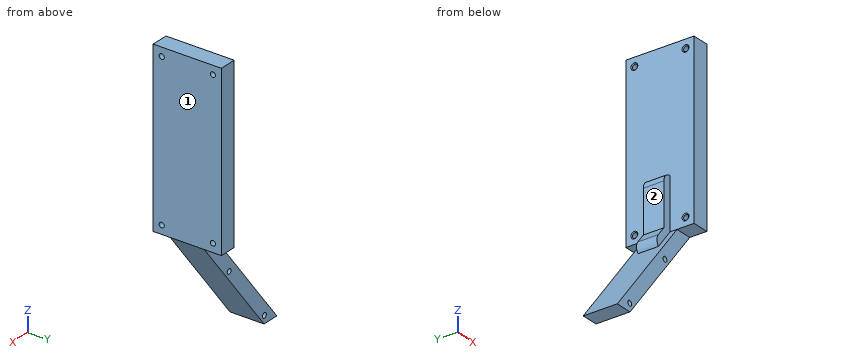
```python
from build123d import *

# Parameters (mm, degrees)
SKETCH_1_W           = 100
SKETCH_1_H           = 40
EXTRUDE_1_DEPTH      = 10
EXTRUDE_2_DEPTH      = 30
SKETCH_4_R           = 1.5
CUT_EXTRUDE_1_DEPTH  = 127.085153879
CUT_EXTRUDE_2_DEPTH  = 10
SKETCH_7_R           = 1.5
CUT_EXTRUDE_3_DEPTH  = 10
CHAMFER_2_SIZE       = 0.5
EXTRUDE_3_DEPTH      = 6
EXTRUDE_3_DEPTH_BACK = 6
FILLET_1_R           = 5


with BuildPart() as part:
    # 草图1 → 凸台-拉伸1 (new body)
    with BuildSketch(Plane(origin=(0, 0, 0), x_dir=(0, 0, -1), z_dir=(1, 0, 0))):
        Rectangle(SKETCH_1_W, SKETCH_1_H)
    extrude(amount=EXTRUDE_1_DEPTH)

    # 草图3 → 凸台-拉伸2 (add)
    with BuildSketch(Plane(origin=(0, 20, 0), x_dir=(1, 0, 0), z_dir=(0, 1, 0))):
        Polygon((10, 50), (-36.87713759, 110), (-46.87713759, 110), (0, 50), align=None)
    extrude(amount=-EXTRUDE_2_DEPTH)

    # 草图4 → 切除-拉伸1 (cut, through all)
    with BuildSketch(Plane(origin=(0, 20, 0), x_dir=(1, 0, 0), z_dir=(0, 1, 0))):
        with Locations(Location((-37.168406916, 105.5, 0), (0, 0, 270))):
            Circle(SKETCH_4_R)
        with Locations(Location((-9.463640527, 70.039516088, 0), (0, 0, 270))):
            Circle(SKETCH_4_R)
    extrude(amount=-CUT_EXTRUDE_1_DEPTH, mode=Mode.SUBTRACT)

    # 草图5 → 切除-拉伸2 (cut)
    with BuildSketch(Plane(origin=(0, 20, 0), x_dir=(1, 0, 0), z_dir=(0, 1, 0))):
        Polygon((10, 50), (0, 50), (-46.87713759, 110), (-36.87713759, 110), align=None)
    extrude(amount=-CUT_EXTRUDE_2_DEPTH, mode=Mode.SUBTRACT)

    # 草图7 → 切除-拉伸3 (cut)
    with BuildSketch(Plane(origin=(10, 0, 0), x_dir=(0, 0, -1), z_dir=(1, 0, 0))):
        with Locations((-45, 15)):
            Circle(SKETCH_7_R)
        with Locations((-45, -15)):
            Circle(SKETCH_7_R)
        with Locations((45, -15)):
            Circle(SKETCH_7_R)
        with Locations((45, 15)):
            Circle(SKETCH_7_R)
    extrude(amount=-CUT_EXTRUDE_3_DEPTH, mode=Mode.SUBTRACT)

    # 倒角2
    chamfer_2_edges = [part.edges().sort_by_distance(p)[0] for p in [
        (0, 15, -43.5),
        (0, -15, -43.5),
        (0, -15, 46.5),
        (0, 15, 46.5),
    ]]
    chamfer(chamfer_2_edges, length=CHAMFER_2_SIZE)

    # 草图9 → 凸台-拉伸3 (add, two sides: drawn at the far end of the back side and taken through both)
    with BuildSketch(Plane(origin=(0, 0, 0), x_dir=(1, 0, 0), z_dir=(0, 1, 0)).offset(-EXTRUDE_3_DEPTH_BACK)):
        Polygon((-9.23492213, 61.820161304), (-12.339726869, 59.394421988), (-5, 50), (-5, 20), (0, 20), (0, 50), align=None)
    extrude(amount=EXTRUDE_3_DEPTH + EXTRUDE_3_DEPTH_BACK)

    # 圆角1
    # the kernel refuses this fillet: 5 mm, written as the material it takes off along each edge
    with BuildSketch(Plane(origin=(-5, -18.5, -20), x_dir=(1, 0, 0), z_dir=(0, 1, 0))) as fillet_1_piece_1:
        with BuildLine():
            CenterArc((FILLET_1_R, FILLET_1_R), FILLET_1_R, 180, 90)
            Line((0, FILLET_1_R), (-FILLET_1_R * 0.02, FILLET_1_R))
            Line((-FILLET_1_R * 0.02, FILLET_1_R), (-FILLET_1_R * 0.02, -FILLET_1_R * 0.02))
            Line((-FILLET_1_R * 0.02, -FILLET_1_R * 0.02), (FILLET_1_R, -FILLET_1_R * 0.02))
            Line((FILLET_1_R, -FILLET_1_R * 0.02), (FILLET_1_R, 0))
        make_face()
    extrude(amount=37, mode=Mode.SUBTRACT)
    with BuildSketch(Plane(origin=(-12.339726869, -18.215899984, -59.394421988), x_dir=(0.7880107536067237, 0, -0.6156614753256561), z_dir=(0, 1, 0))) as fillet_1_piece_2:
        with BuildLine():
            CenterArc((5, -4.886359993), FILLET_1_R, 102.23895269, 77.76104731)
            Line((0, -4.886359993), (-0.1, -4.886359993))
            Line((-0.1, -4.886359993), (-0.1, 0))
            Line((-0.1, 0), (0, 0.1))
            ThreePointArc((0, 0.1), (1.970026884, 0.1), (3.918854843, 0.0977272))
            Line((3.918854843, 0.0977272), (3.940053768, 0))
        make_face()
    extrude(amount=36.431799967, mode=Mode.SUBTRACT)


solid = part.part
```
Verification items for the finished model (mm, model axes). Face numbers are marked on the shaded views. A direction names the side the tool comes from. Coordinates: 2 decimals unless noted, no trailing zeros. Order: outer loops, then holes, each group sorted by start corner. A loop starts at its lowest first (then second) coordinate and runs counter-clockwise, first axis right, second up. Notation, with made-up numbers: (7.5, 2) -> (51.5, 2) arc R29 ccw to (51.5, 23) -> close; hole circle Ø1 at (-8, 54). An arc over 180 degrees is marked (long way). Put each result on its own line as item: value. Start each with the question number.
1) Tool access check on the marked faces 1 and 2. Record the directions out of +Z, -Z, +X, -X, +Y, -Y that give a thin tool (end or side, any length) a straight path to the whole face; none if there is none.
2) Material ranges on L1, parallel to Y at x = 3, z = -45; L2, parallel to Z at x = 7.5, y = 10.5; L3, parallel to X at y = -2.5, z = -45.5, recorded low to high.
3) Cross-section at A-A (y = -15). Enter the section's corners in (x, z), plus the area to 4 significant figures.
4) Cross-section at D-D (z = -105.5). Enter the section's corners in (x, y), plus the area to 3 significant figures.
5) Go/stop test with flat-tipped pins: pin 1 (5 mm diameter, centred on y = -15, z = 45, fed in from -X); pin 2 (8 mm diameter, centred on x = -20.5, y = -6.5, fed in from -Z); pin 3 (3 mm diameter, centred on x = 4.5, y = 16, fed in from -Z); pin 4 (12 mm diameter, centred on x = -5.5, y = -1, fed in from +Z). Record where each tip stops, or that it passes through.
6) Cross-section at C-C (x = 2). Enter the section's corners in (y, z).
7) Cross-section at B-B (z = 45). Enter the section's corners in (x, y).
Geometry check:
1. face 1: +Z, -Z, +X, +Y, -Y
1. face 2: +Z, -X, +Y, -Y
2. L1: y = -20 to -16.5, -13.5 to 13.5, 16.5 to 20
2. L2: z = -50 to 50
2. L3: x = -5 to 10
3. outline: (0, -50) -> (10, -50) -> (10, -46.5) -> (0.5, -46.5) -> (0, -47) -> close; (0, -43) -> (0.5, -43.5) -> (10, -43.5) -> (10, 43.5) -> (0.5, 43.5) -> (0, 43) -> close; (0, 47) -> (0.5, 46.5) -> (10, 46.5) -> (10, 50) -> (0, 50) -> close
3. area: 939.5 mm^2
4. outline: (-43.36, -10) -> (-38.67, -10) -> (-38.67, 10) -> (-43.36, 10) -> close; (-35.67, -10) -> (-33.36, -10) -> (-33.36, 10) -> (-35.67, 10) -> close
4. area: 140 mm^2
5. pin 1: stops at x = 0
5. pin 2: stops at z = -94.16
5. pin 3: stops at z = -50
5. pin 4: stops at z = 50
6. outline: (-20, -50) -> (-10, -50) -> (-10, -60.24) -> (10, -60.24) -> (10, -50) -> (20, -50) -> (20, 50) -> (-20, 50) -> close; hole circle Ø3 at (-15, -45); hole circle Ø3 at (-15, 45); hole circle Ø3 at (15, -45); hole circle Ø3 at (15, 45)
7. outline: (0, -20) -> (10, -20) -> (10, -16.5) -> (0.5, -16.5) -> (0, -17) -> close; (0, -13) -> (0.5, -13.5) -> (10, -13.5) -> (10, 13.5) -> (0.5, 13.5) -> (0, 13) -> close; (0, 17) -> (0.5, 16.5) -> (10, 16.5) -> (10, 20) -> (0, 20) -> close
